Could you check a few things on this drawing? It's one solid part, dimensions in mm from its lowest x, y, z. A direction names the side the tool comes from. Give positions to 0.01 mm unless a question says otherwise; leave off trailing zeros. Loops run counter-clockwise (first coordinate to the right, second up) from the corner with the lowest first, then second, coordinate; pieces in that order, holes last. Notation, with made-up numbers: (87.25, 34.25) - (98.25, 34.25) arc R24 cw to (98.25, 72.25) - close; hole circle Ø1 at (36.5, 38). An arc over 180 degrees is marked (long way). Answer as a JSON object with one key per item and string values.
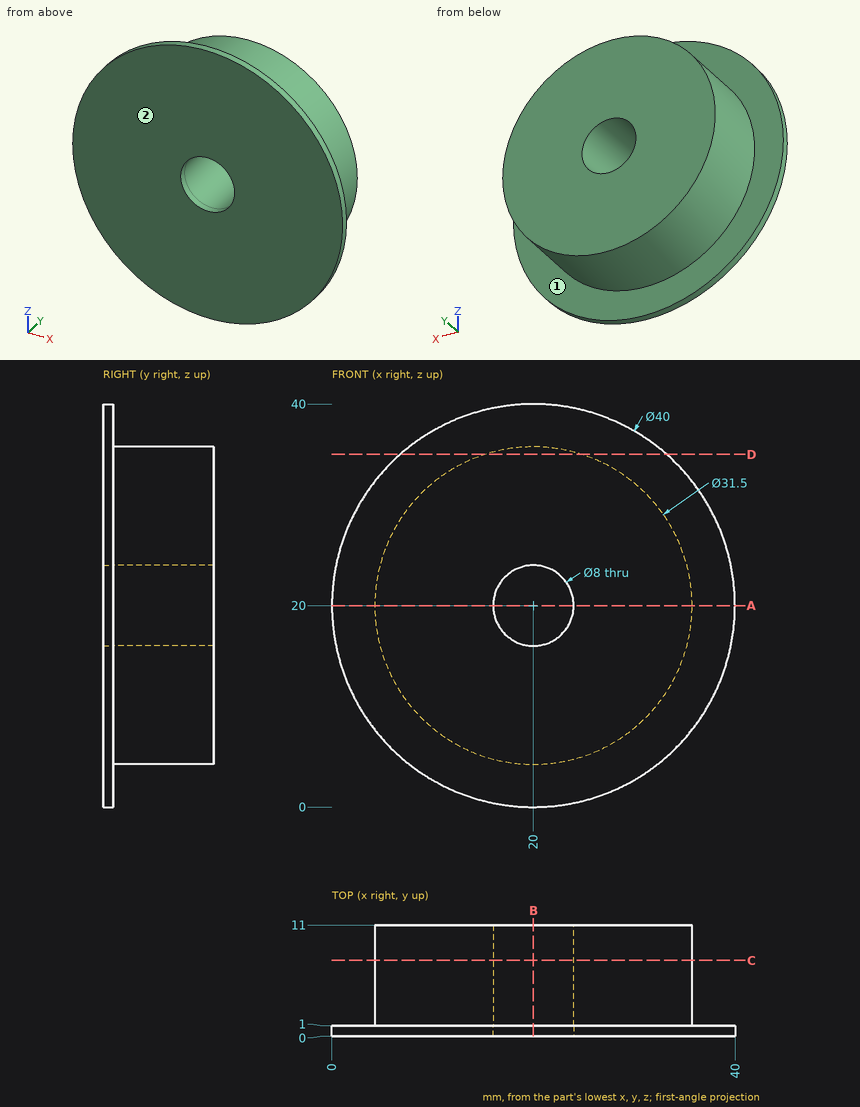
1) Imagine slicing it at A-A on z = 20. Write out the boundary of the cut face in (x, y).
Check sheet entries:
{"outline": "(0, 0) - (16, 0) - (16, 11) - (4.25, 11) - (4.25, 1) - (0, 1) - close; (24, 0) - (40, 0) - (40, 1) - (35.75, 1) - (35.75, 11) - (24, 11) - close"}
2) I need wall thicknesses on L1, parallel to Z at x = 20, y = 0.3; L2, parallel to Z at x = 20, y = 4.25; L3, parallel to Y at x = 12, z = 2. Which ranges of each line are inside material? Lowest first, please.
Check sheet entries:
{"L1": "0 to 16, 24 to 40", "L2": "4.25 to 16, 24 to 35.75", "L3": "0 to 1"}
3) Imagine slicing it at C-C on y = 7.5. Write out the boundary of the cut face in (x, z).
Check sheet entries:
{"outline": "circle Ø31.5 at (20, 20); hole circle Ø8 at (20, 20)"}
4) Imagine slicing it at B-B on x = 20. Write out the boundary of the cut face in (y, z).
Check sheet entries:
{"outline": "(0, 0) - (1, 0) - (1, 4.25) - (11, 4.25) - (11, 16) - (0, 16) - close; (0, 24) - (11, 24) - (11, 35.75) - (1, 35.75) - (1, 40) - (0, 40) - close"}
5) Which directions (+Z, -Z, +X, -X, +Y, -Y) give clear straight access to the entire face, cutting with the end or side of a thin tool? Please do the marked faces 1 and 2.
Check sheet entries:
{"face 1": "+Y", "face 2": "+Z, -Z, +X, -X, -Y"}
6) I'm going to push flat-ended pins straight in: P1, Ø1, axis at y = 6.5, z = 17.5, coming from the -X side; P2, Ø3, axis at x = 11, y = 2, coming from the -Z side; P3, Ø6, axis at y = 2, z = 10, coming from the +X side. Where does each tip first touch, or does it pass through?
Check sheet entries:
{"P1": "x = 4.38", "P2": "z = 1.62", "P3": "x = 38.67"}
7) Imagine slicing it at D-D on z = 35. Write out the boundary of the cut face in (x, y), and give its area (3 significant figures).
Check sheet entries:
{"outline": "(6.77, 0) - (33.23, 0) - (33.23, 1) - (24.8, 1) - (24.8, 11) - (15.2, 11) - (15.2, 1) - (6.77, 1) - close", "area": "123 mm2"}
